For this review, take the finished solid that the model builds, in its own axes (mm). A direction names the side the tool comes from. Coordinates: 2 decimals unless noted, no trailing zeros. Write each loop counter-clockwise with the first axis right and the second up, starting at its lowest first coordinate (ties: lowest second). Pieces come first, ordered by that corner, then holes. Notation, with made-up numbers: M -20.75,53.25 L 37.25,53.25 A13 ccw 37.25,60.25 Z; hole C 14,-16 d9. An arc over 180 degrees is marked long. Return JSON: item names as keys, results as strings.
Autodesk Inventor part; units mm, degrees
ref_plane "XY Plane" through (0, 0, 0) normal (0, 0, 1) x (1, 0, 0)
sketch "Sketch1" plane through (0, 0, 0) normal (0, 0, 1) x (1, 0, 0)
  arc A0 (20.8333, 123.2517) -> (-20.8333, 123.2517) centre (0, 0) ccw
  arc A1 (20, 118.3216) -> (-20, 118.3216) centre (0, 0) ccw
  line L0 (0, 0) -> (0, 143.8844) construction
  line L1 (-20, 118.3216) -> (-20.8333, 123.2517)
  line L2 (20, 118.3216) -> (20.8333, 123.2517)
  dimension "d0" = 250
  dimension "d1" = 5
  dimension "d2" = 40
extrude "Extrusion1" add sketch "Sketch1" along normal mid plane 40
ref_plane "Work Plane1" through (0, 120, 0) normal (0, 1, 0) x (-1, 0, 0)
sketch "Sketch2" plane through (0, 120, 0) normal (0, 1, 0) x (-1, 0, 0)
  circle A0 centre (0, 0) radius 5
  point P0 (0, 0)
  dimension "d5" = 10
extrude "Extrusion2" add sketch "Sketch2" along normal blind 35
ref_plane "Work Plane2" through (-5, 120, 0) normal (1, 0, 0) x (0, 1, 0)
sketch "Sketch3" plane through (-5, 120, 0) normal (1, 0, 0) x (0, 1, 0)
  circle A0 centre (30, 0) radius 1.8
  line L0 (35, -5) -> (35, 5)
  line L1 (-151, 0) -> (66, 0)
  point P0 (-120, 0)
  dimension "d8" = 3.6
  dimension "d9" = 5
extrude "Extrusion3" cut sketch "Sketch3" along normal blind 5
chamfer "Chamfer1" distance 0.5 angle 45 2 edges at (-4.6648, 149.9993, -1.8) (-4.6648, 150.0007, 1.8)
properties part number "shiftt_fixed_plate2"
1. We need section C-C (x = -13.5). State the section outline as (y, z) points, plus the area to 3 significant figures.
Checks:
{"outline": "M 119.24,-20 L 124.27,-20 L 124.27,20 L 119.24,20 Z", "area": "201 mm2"}
2. Clearance check with flat-ended pins moving along their axes: pin 1 Ø5 at (y, z) = (148.5, 0.5) entering from -X; pin 2 Ø1.8 at (y, z) = (149.5, -1) entering from -X; pin 3 Ø10 at (y, z) = (135, -6) entering from +X; pin 4 Ø1 at (y, z) = (145.5, -6) entering from -X. State where each tip first meets the part, or that it passes through.
Checks:
{"pin 1": "x = -5", "pin 2": "x = -4.42", "pin 3": "x = 4.9", "pin 4": "through"}
3. We need section A-A (z = -8.5). State the section outline as (x, y) points, plus the area to 3 significant figures.
Checks:
{"outline": "M -20.83,123.25 L -20,118.32 A120 cw 20,118.32 L 20.83,123.25 A125 ccw Z", "area": "205 mm2"}
4. Draft analysis for pull direction Z (two halves, no side actions). For faces 1 (the face through (20.41, 120.75, -0.28)), 2 (the face through (-2.28, 148.2, -0.08)), 3 (the face through (0, 122, -20)), state which applies: +Z half, -Z half, draft (parallel to the pull), parting line (faces both ways), or undercut.
Checks:
{"face 1": "draft", "face 2": "undercut", "face 3": "-Z half"}
5. Wall thickness on L1, parallel to Z at x = -1.2, y = 150; L2, parallel to Y at x = -1.4, z = 0; L3, parallel to Y at x = 0, z = -2.5: over which ranges is each line inside the solid? List them lowest first. Write a range as from..to.
Checks:
{"L1": "-4.85..-1.8, 1.8..4.85", "L2": "119.99..148.2, 151.8..155", "L3": "120..155"}
6. For faces 4 (the face through (-4.943, 124.902, 4.164)), 5 (the face through (0, 122, 20)), 6 (the face through (0, 150, 0)), list the 3-axis set-ups (+Z, -Z, +X, -X, +Y, -Y) from which the entire face can be reached by the end or side of a thin tool; tool diameter is ignored.
Checks:
{"face 4": "+Y", "face 5": "+Z, +X, -X, +Y, -Y", "face 6": "-X"}
7. We need section B-B (y = 144). State the section outline as (x, z) points.
Checks:
{"outline": "C 0,0 d10"}
